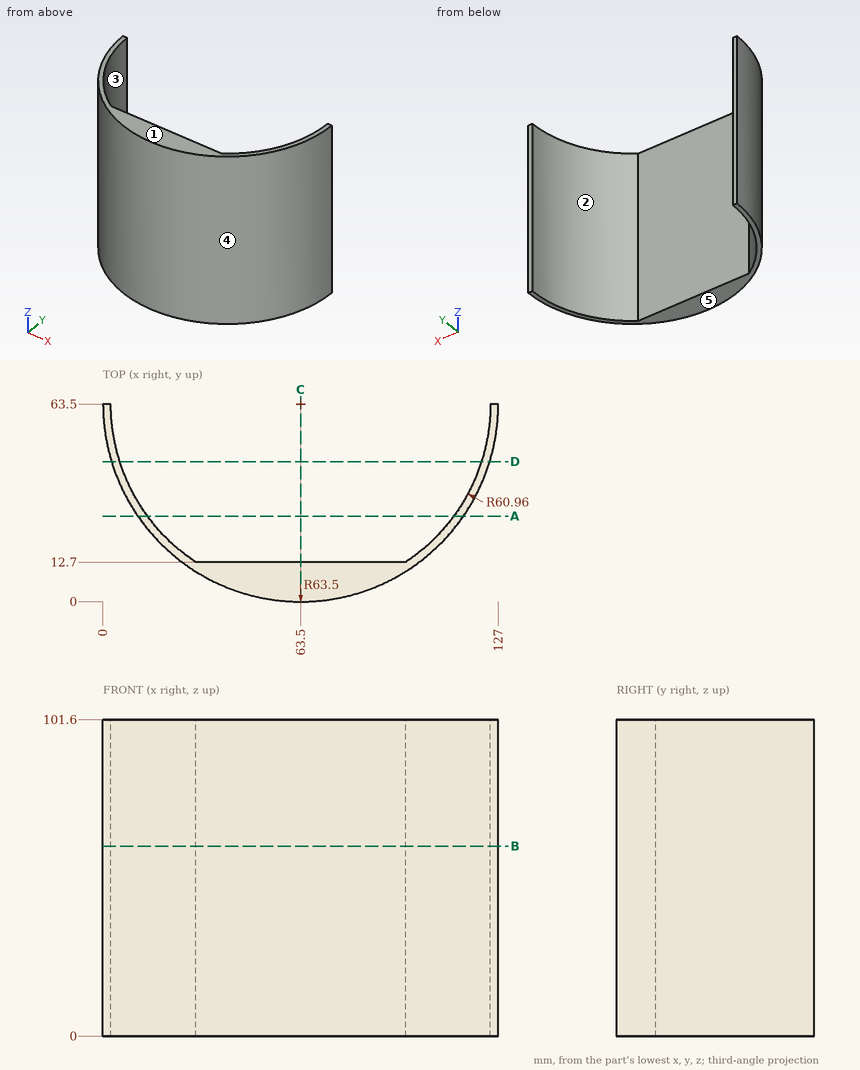
The figure shows three views and two pictorial views of one solid part (mm, origin at its lowest corner). Answer the questions. A direction names the side the tool comes from. Round coordinates to 2 decimals unless told otherwise and drop trailing zeros. Loops run counter-clockwise (first coordinate to the right, second up) from the corner with the lowest first, then second, coordinate; pieces in that order, holes last. Notation, with made-up numbers: (84, -27.75) - (109, -27.75) arc R35 ccw to (109, 9.25) - close; hole circle Ø10 at (-33, 53.25). An arc over 180 degrees is marked (long way). One line per question, with ' | ' between items. Start each with the question number.
Q1. For the marked faces 1 and 2, determine the directions among +Z, -Z, +X, -X, +Y, -Y from which every point of the face is accessible in a straight line to the end or side of a thin tool.
Q2. Section A-A on y = 27.5 is taken. Give the vertices of the cut face in (x, z), plus the area to 3 significant figures.
Q3. For a pull along X with two mould halves and no side action, classify the marked faces 3, 4 and 5 as +X half, -X half, draft (parallel to the pull), parting line (faces both ways), or undercut.
Q4. Section C-C on x = 63.5 is taken. Give the vertices of the cut face in (y, z).
Q5. Flat-ended cylindrical pins translate along their axes: pin 1 (6 mm diameter, centred on x = 19, z = 35.5, fed in from -Y); pin 2 (1 mm diameter, centred on y = 8.5, z = 14, fed in from +X); pin 3 (6 mm diameter, centred on x = 53.5, z = 47, fed in from -Y). Find the tip coordinate at first contact, or state that the pin passes through.
Q6. Section B-B on z = 61 is taken. Give the vertices of the cut face in (x, y), plus the area to 3 significant figures.
Q7. Find the intervals of material crossed by L1, parallel to X at y = 51.5, z = 55; L2, parallel to X at y = 38.5, z = 60.5; L3, parallel to Y at x = 40, z = 9.5, in increasing order.
Q8. Section D-D on y = 45 is taken. Give the vertices of the cut face in (x, z), plus the area to 3 significant figures.
Established:
1) face 1: +Z, +X, -X, +Y, -Y | face 2: +Z, -Z, +Y
2) outline: (11.19, 0) - (14.31, 0) - (14.31, 101.6) - (11.19, 101.6) - close; (112.69, 0) - (115.81, 0) - (115.81, 101.6) - (112.69, 101.6) - close | area: 633 mm²
3) face 3: undercut | face 4: parting line | face 5: draft
4) outline: (0, 0) - (12.7, 0) - (12.7, 101.6) - (0, 101.6) - close
5) pin 1: y = 15.44 | pin 2: x = 96.09 | pin 3: y = 0.39
6) outline: (0, 63.5) arc R63.5 ccw to (127, 63.5) - (124.46, 63.5) arc R60.96 cw to (97.2, 12.7) - (29.8, 12.7) arc R60.96 cw to (2.54, 63.5) - close | area: 961 mm²
7) L1: 1.14 to 3.73, 123.27 to 125.86 | L2: 5.13 to 7.9, 119.1 to 121.87 | L3: 4.51 to 12.7
8) outline: (2.75, 0) - (5.41, 0) - (5.41, 101.6) - (2.75, 101.6) - close; (121.59, 0) - (124.25, 0) - (124.25, 101.6) - (121.59, 101.6) - close | area: 541 mm²
